from build123d import *

# Parameters (mm, degrees)
EXTRUDE_1_DEPTH     = 2.5
SKETCH_5_R          = 0.6
CUT_EXTRUDE_1_DEPTH = 19.036421485
CUT_EXTRUDE_START   = -2
SKETCH_5_3_R        = 1
CUT_EXTRUDE_2_DEPTH = 1


with BuildPart() as part:
    # 草图4 → 凸台-拉伸1 (new body)
    with BuildSketch(Plane.XY):
        Polygon((8.5, -1.5), (17.75, -1.5), (17.75, -3.5), (-4.5, -3.5), (-4.5, -1.5), (-0.5, 0), (0, 0), (0, -1.5), (4, -1.5), (4, 0), (4.5, 0), align=None)
    extrude(amount=EXTRUDE_1_DEPTH)

    # 草图5 → 切除-拉伸1 (cut, through all)
    with BuildSketch(Plane(origin=(0, -1.5, 0), x_dir=(1, 0, 0), z_dir=(0, 1, 0))):
        with Locations(Location((2, -1.25, 0), (0, 0, 270))):
            Circle(SKETCH_5_R)
    extrude(amount=-CUT_EXTRUDE_1_DEPTH, mode=Mode.SUBTRACT)

    # 草图5<3> → 切除-拉伸2 (cut)
    with BuildSketch(Plane(origin=(0, -1.5, 0), x_dir=(1, 0, 0), z_dir=(0, 1, 0)).offset(CUT_EXTRUDE_START)):
        with Locations((2, -1.25)):
            Circle(SKETCH_5_3_R)
    extrude(amount=CUT_EXTRUDE_2_DEPTH, mode=Mode.SUBTRACT)

    # 镜向1: part across plane


with BuildPart() as part_1:
    add(part.part)
    add(part.part.mirror(Plane.XY.offset(2.5)))

    # 镜向2: part across plane


with BuildPart() as part_2:
    add(part_1.part)
    add(part_1.part.mirror(Plane(origin=(17.75, 0, 2.5), x_dir=(0, 0, 1), z_dir=(1, 0, 0))))


solid = part_2.part
Could you check a few things on this model? Use its own coordinates, in mm. A direction names the side the tool comes from. Round coordinates to 2 decimals unless told otherwise and drop trailing zeros. Order: outer loops, then holes, each group sorted by start corner. A loop starts at its lowest first (then second) coordinate and runs counter-clockwise, first axis right, second up. Notation, with made-up numbers: M 1.5,20.5 L 22.5,20.5 A35 ccw 22.5,54.5 Z; hole C -12.5,54 d1. An arc over 180 degrees is marked long. One line per item, written item: value.
(1) I'm going to push flat-ended pins straight in: P1, Ø1.8, axis at x = 2, z = 1.25, coming from the -Y side; P2, Ø2, axis at x = 2, z = 3.5, coming from the -Y side; P3, Ø1.4, axis at x = 33.5, z = 3.75, coming from the +Y side; P4, Ø1.1, axis at x = 33.5, z = 1.25, coming from the -Y side. Where does each tip first touch, or does it pass through?
Ans:
P1: stops at y = -2.5
P2: stops at y = -3.5
P3: stops at y = -1.5
P4: passes through
(2) I need wall thicknesses on line 1 along Z through (x, y) = (33.5, -3.2); line 2 along Z through (x, y) = (33.5, -1.7); line 3 along X through (y, z) = (-3.3, 1.25). Which ranges of each line are inside material? Lowest first, please. Write a range as from..to.
Ans:
line 1: z = 0..0.25, 2.25..2.75, 4.75..5
line 2: z = 0..0.65, 1.85..3.15, 4.35..5
line 3: x = -4.5..1, 3..32.5, 34.5..40
(3) Imagine slicing it at A-A (z = 3.75). Count the separate pieces of the cut face and the enclosed holes in it, and give its area (3 significant figures).
Ans:
separate pieces: 3
enclosed holes: 0
area: 97.6 mm^2
(4) Imagine slicing it at D-D (x = 7.5). Write out the boundary of the cut face in (y, z) (3 decimals).
Ans:
outline: M -3.5,0 L -1.125,0 L -1.125,5 L -3.5,5 Z
(5) Imagine slicing it at C-C (x = 23). Write out the boundary of the cut face in (y, z), and give its area (3 significant figures).
Ans:
outline: M -3.5,0 L -1.5,0 L -1.5,5 L -3.5,5 Z
area: 10.0 mm^2
(6) Imagine slicing it at B-B (x = 33.5). Write out the boundary of the cut face in (y, z), and give its area (3 significant figures).
Ans:
outline: M -3.5,0 L -1.5,0 L -1.5,0.65 L -2.5,0.65 L -2.5,0.25 L -3.5,0.25 Z; M -3.5,2.25 L -2.5,2.25 L -2.5,1.85 L -1.5,1.85 L -1.5,3.15 L -2.5,3.15 L -2.5,2.75 L -3.5,2.75 Z; M -3.5,4.75 L -2.5,4.75 L -2.5,4.35 L -1.5,4.35 L -1.5,5 L -3.5,5 Z
area: 3.60 mm^2
(7) If we mould it in two halves opening along X, with no side actions, what happens to faces 1 (the flat face through (-4.5, -3, 3)), 2 (the flat face through (38.03, -0.76, 2.54)), 3 (the cylindrical face through (32.546, -3.007, 0.95))? For each: released by +X, released by -X, zero draft, split by the parting line, or undercut.
Ans:
face 1: released by -X
face 2: released by +X
face 3: undercut
(8) Which directions (+Z, -Z, +X, -X, +Y, -Y) give clear straight access to the entire face, cutting with the end or side of a thin tool? Please do faces 4 (the cylindrical face through (2.506, -1.993, 1.573)), 5 (the flat face through (18, -1.5, 3)), 6 (the cylindrical face through (1.263, -3.007, 4.426)).
Ans:
face 4: +Y, -Y
face 5: +Z, -Z, +Y
face 6: -Y
